from build123d import *

# Parameters (mm, degrees)
SKETCH1_R                 = 3
CRANK_BODY_DEPTH          = 10
SKETCH2_R                 = 1.55
DOWEL_SHAFT_DEPTH         = 9
PIN_SHAFT_BODY_DEPTH      = 3
PIN_SHAFT_BODY_DEPTH_BACK = 3
SKETCH4_R                 = 2.5
PIN_SHAFT_DEPTH           = 7
SKETCH1_2_OUTSIDE_W       = 12.286
SKETCH1_2_OUTSIDE_H       = 15.286
SKETCH1_2_OUTSIDE_R       = 3
SMOOTHING_CUTS_DEPTH      = 10.5


with BuildPart() as part:
    # Sketch1 → crank_body (new body)
    with BuildSketch(Plane(origin=(0, 0, 0), x_dir=(1, 0, 0), z_dir=(0, 1, 0))):
        Circle(SKETCH1_R)
    extrude(amount=CRANK_BODY_DEPTH)

    # Sketch2 → dowel_shaft (cut)
    with BuildSketch(Plane.XZ):
        Circle(SKETCH2_R)
    extrude(amount=-DOWEL_SHAFT_DEPTH, mode=Mode.SUBTRACT)

    # Sketch3 → pin_shaft_body (add, two sides)
    with BuildSketch(Plane(origin=(0, 0, 0), x_dir=(0, 0, -1), z_dir=(1, 0, 0))) as pin_shaft_body_sk:
        with BuildLine():
            Line((-3, 10.5), (-3, 10))
            Line((-3, 10), (3, 10))
            Line((3, 10), (3, 10.5))
            Line((3, 10.5), (2.828427125, 10.5))
            ThreePointArc((2.828427125, 10.5), (0, 18.5), (-2.828427125, 10.5))
            Line((-2.828427125, 10.5), (-3, 10.5))
        make_face()
    extrude(amount=PIN_SHAFT_BODY_DEPTH)
    extrude(pin_shaft_body_sk.sketch, amount=-PIN_SHAFT_BODY_DEPTH_BACK)

    # Sketch4 → pin_shaft (cut, through all)
    with BuildSketch(Plane(origin=(3, 0, 0), x_dir=(0, 0, -1), z_dir=(1, 0, 0))):
        with Locations((0, 14)):
            Circle(SKETCH4_R)
    extrude(amount=-PIN_SHAFT_DEPTH, mode=Mode.SUBTRACT)

    # Sketch1_2 outside → smoothing_cuts (cut)
    with BuildSketch(Plane(origin=(0, 0, 0), x_dir=(1, 0, 0), z_dir=(0, 1, 0))):
        Rectangle(SKETCH1_2_OUTSIDE_W, SKETCH1_2_OUTSIDE_H)
        Circle(SKETCH1_2_OUTSIDE_R, mode=Mode.SUBTRACT)
    extrude(amount=SMOOTHING_CUTS_DEPTH, mode=Mode.SUBTRACT)


solid = part.part
Read the model definition and answer for the solid it produces. Units are mm, in the model's axes. A direction names the side the tool comes from. Round coordinates to 2 decimals unless told otherwise and drop trailing zeros. Write each loop counter-clockwise with the first axis right and the second up, starting at its lowest first coordinate (ties: lowest second). Pieces come first, ordered by that corner, then holes.
1. The part is cut by section A-A, the plane x = 0. Determine the outline of the cut face in (y, z).
2. The part is cut by section B-B, the plane y = 14. Determine the outline of the cut face in (x, z), then the cut area to 3 significant figures.
3. Straight lines are drawn through the part: L1, parallel to Y at x = 1.45, z = 0; L2, parallel to Z at x = 0, y = 5.25; L3, parallel to Z at x = -1.05, y = 16.25. For each, find the intervals that lie inside material, in ascending order.
4. The part is cut by section C-C, the plane y = 17.5. Determine the outline of the cut face in (x, z), then the cut area to 3 significant figures.
5. Given pin 1 Ø1 at (x, z) = (2.5, 1) entering from -Y; pin 2 Ø1 at (x, z) = (0.5, 0) entering from -Y, each flat-ended and moving along its own axis, determine where each tip first touches the part or whether it passes through.
6. The part is cut by section D-D, the plane x = -2.5. Determine the outline of the cut face in (y, z).
7. Determine the mould class of faces 4 (the face through (0.715, 4.437, -1.375)), 5 (the face through (3, 16, -2)), 6 (the face through (0.04, 11.56, 0.54)) for opening direction X: pulls with the +X half, pulls with the -X half, needs draft (parallel to the pull), parting line crosses it, or undercut.
8. Which of the six approach directions +Z, -Z, +X, -X, +Y, -Y give full straight-line access (tool end or side, diameter ignored) to faces 1 (the face through (2.4, 10.5, 2.2)), 2 (the face through (-2.5, 10.5, -2.2)), 3 (the face through (-2.4, 10.5, 2.2))?
Values:
1. outline: (0, -3) - (10.5, -3) - (10.5, -2.83) arc R4.5 ccw (long way) to (10.5, 2.83) - (10.5, 3) - (0, 3) - (0, 1.55) - (9, 1.55) - (9, -1.55) - (0, -1.55) - close; hole circle Ø5 at (14, 0)
2. outline: (-3, -4.5) - (3, -4.5) - (3, -2.5) - (-3, -2.5) - close; (-3, 2.5) - (3, 2.5) - (3, 4.5) - (-3, 4.5) - close
2. area: 24.0 mm2
3. L1: y = 9 to 11.5, 16.5 to 18.5
3. L2: z = -3 to -1.55, 1.55 to 3
3. L3: z = -3.9 to -1.09, 1.09 to 3.9
4. outline: (-3, -2.83) - (3, -2.83) - (3, 2.83) - (-3, 2.83) - close
4. area: 33.9 mm2
5. pin 1: stops at y = 0
5. pin 2: stops at y = 9
6. outline: (0, -1.66) - (10.5, -1.66) - (10.5, -2.83) arc R4.5 ccw (long way) to (10.5, 2.83) - (10.5, 1.66) - (0, 1.66) - close; hole circle Ø5 at (14, 0)
7. face 4: undercut
7. face 5: pulls with the +X half
7. face 6: needs draft
8. face 1: +Z, +X, -Y
8. face 2: -Z, -X, -Y
8. face 3: +Z, -X, -Y
